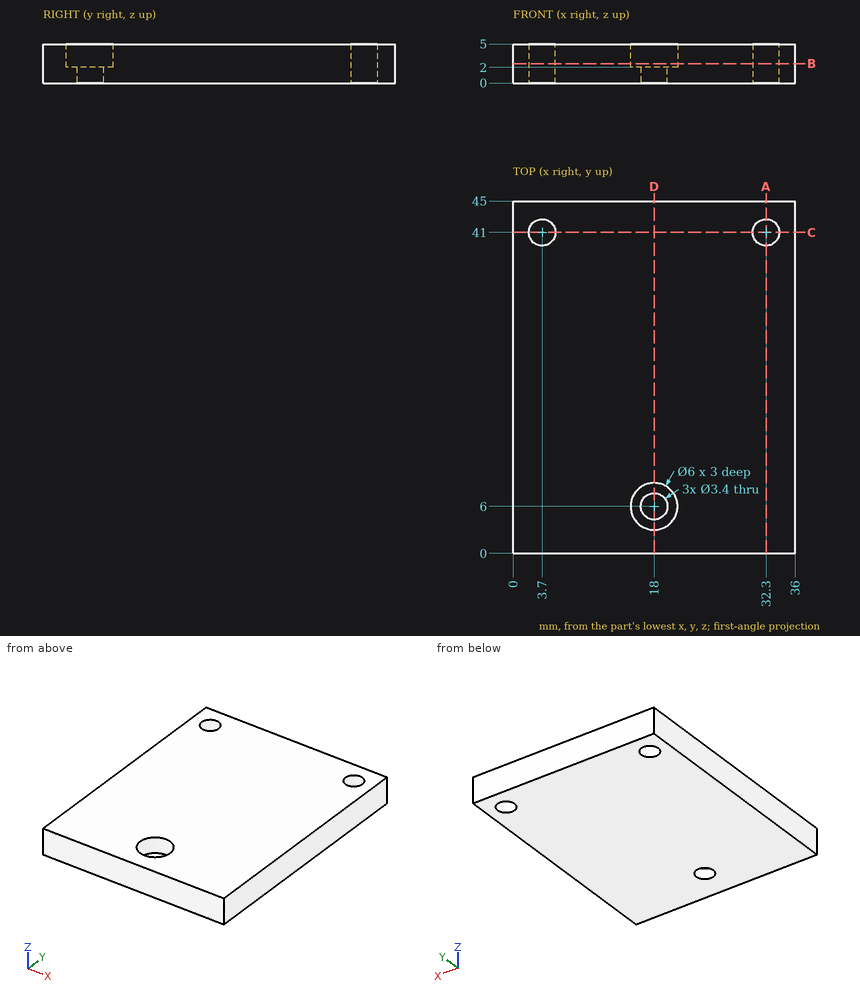
The figure shows three views and two pictorial views of one solid part (mm, origin at its lowest corner). Answer the questions. Coordinates: 2 decimals unless noted, no trailing zeros. Loops run counter-clockwise (first coordinate to the right, second up) from the corner with the lowest first, then second, coordinate; pieces in that order, holes last.
(1) Consider line 1 along X through (y, z) = (41, 3.95); line 2 along X through (y, z) = (6, 0.55); line 3 along Y through (x, z) = (32.3, 2.05). Determine where each line is inside the solid, lowest interval first.
Solution:
line 1: x = 0 to 2, 5.4 to 30.6, 34 to 36
line 2: x = 0 to 16.3, 19.7 to 36
line 3: y = 0 to 39.3, 42.7 to 45
(2) A flat-ended cylindrical pin translates along its axis: pin 1 Ø3 at (x, y) = (19.5, 7.5) entering from +Z. Find the tip coordinate at first contact, or state that the pin passes through.
Solution:
pin 1: stops at z = 5
(3) The part is cut by section B-B (z = 2.5). Determine the outline of the cut face in (x, y), and give its area (3 significant figures).
Solution:
outline: (0, 0) - (36, 0) - (36, 45) - (0, 45) - close; hole circle Ø3.4 at (3.7, 41); hole circle Ø6 at (18, 6); hole circle Ø3.4 at (32.3, 41)
area: 1,570 mm2
(4) The part is cut by section C-C (y = 41). Determine the outline of the cut face in (x, z).
Solution:
outline: (0, 0) - (2, 0) - (2, 5) - (0, 5) - close; (5.4, 0) - (30.6, 0) - (30.6, 5) - (5.4, 5) - close; (34, 0) - (36, 0) - (36, 5) - (34, 5) - close
(5) The part is cut by section D-D (x = 18). Determine the outline of the cut face in (y, z).
Solution:
outline: (0, 0) - (4.3, 0) - (4.3, 2) - (3, 2) - (3, 5) - (0, 5) - close; (7.7, 0) - (45, 0) - (45, 5) - (9, 5) - (9, 2) - (7.7, 2) - close
(6) The part is cut by section A-A (x = 32.3). Determine the outline of the cut face in (y, z).
Solution:
outline: (0, 0) - (39.3, 0) - (39.3, 5) - (0, 5) - close; (42.7, 0) - (45, 0) - (45, 5) - (42.7, 5) - close
